Here's how the part is built. I have some questions about the finished solid (model axes, mm). A direction names the side the tool comes from. Give positions to 0.01 mm unless a question says otherwise; leave off trailing zeros. Order: outer loops, then holes, each group sorted by start corner. A loop starts at its lowest first (then second) coordinate and runs counter-clockwise, first axis right, second up.
from build123d import *

# Parameters (mm, degrees)
F0_R      = 3.1
F0_W      = 5.4
F0_H      = 6
F0_W_2    = 6
F0_H_2    = 5.4
F1_DEPTH  = 6
F2_DEPTH  = 10
F3_R      = 2
F4_SIZE   = 3.5
F1_FACE_R = 6.6
F5_DEPTH  = 2


with BuildPart() as f1:
    # F0 (on Top) → F1 (new body)
    with BuildSketch(Plane.XY):
        Polygon((-7.995946, 7.05), (-7.995946, 0), (-0.945946, 0), (-0.945946, 5.4), (5.054054, 5.4), (5.054054, 0), (12.104054, 0), (12.104054, 7.05), (6.704054, 7.05), (6.704054, 13.05), (12.104054, 13.05), (12.104054, 20.1), (5.054054, 20.1), (5.054054, 14.7), (-0.945946, 14.7), (-0.945946, 20.1), (-7.995946, 20.1), (-7.995946, 13.05), (-2.595946, 13.05), (-2.595946, 7.05), align=None)
        with Locations((2.054054, 10.05)):
            Circle(F0_R, mode=Mode.SUBTRACT)
        with Locations((9.404054, 10.05)):
            Rectangle(F0_W, F0_H)
        with Locations((-5.295946, 10.05)):
            Rectangle(F0_W, F0_H)
        with Locations((2.054054, 17.4)):
            Rectangle(F0_W_2, F0_H_2)
        with Locations((2.054054, 2.7)):
            Rectangle(F0_W_2, F0_H_2)
    extrude(amount=F1_DEPTH)

    # F0 (on Top) → F2 (join)
    with BuildSketch(Plane.XY):
        with Locations((2.054054, 17.4)):
            Rectangle(F0_W_2, F0_H_2)
        with Locations((-5.295946, 10.05)):
            Rectangle(F0_W, F0_H)
        with Locations((2.054054, 2.7)):
            Rectangle(F0_W_2, F0_H_2)
        with Locations((9.404054, 10.05)):
            Rectangle(F0_W, F0_H)
    extrude(amount=F2_DEPTH)

    # F3
    f3_edges = [f1.edges().sort_by_distance(p)[0] for p in [
        (-7.995946, 0, 3),
        (12.104054, 0, 3),
        (12.104054, 20.1, 3),
        (-7.995946, 20.1, 3),
    ]]
    fillet(f3_edges, radius=F3_R)

    # F4
    f4_edges = [f1.edges().sort_by_distance(p)[0] for p in [
        (-1.045946, 10.05, 0),
    ]]
    chamfer(f4_edges, length=F4_SIZE)

    # F1_face (on face) → F5 (join)
    with BuildSketch(Plane(origin=(2.054054, 10.05, 0), x_dir=(1, 0, 0), z_dir=(0, 0, -1))):
        with BuildLine():
            Line((-8.05, -10.05), (8.05, -10.05))
            ThreePointArc((8.05, -10.05), (9.464214, -9.464214), (10.05, -8.05))
            Line((10.05, -8.05), (10.05, 8.05))
            ThreePointArc((10.05, 8.05), (9.464214, 9.464214), (8.05, 10.05))
            Line((8.05, 10.05), (-8.05, 10.05))
            ThreePointArc((-8.05, 10.05), (-9.464214, 9.464214), (-10.05, 8.05))
            Line((-10.05, 8.05), (-10.05, -8.05))
            ThreePointArc((-10.05, -8.05), (-9.464214, -9.464214), (-8.05, -10.05))
        make_face()
        Circle(F1_FACE_R, mode=Mode.SUBTRACT)
    extrude(amount=F5_DEPTH)


solid = f1.part
Q1. I'm going to push flat-ended pins straight in: P1, Ø1.5, axis at x = 7, z = 7, coming from the -Y side; P2, Ø7, axis at x = 2.05, y = 10.05, coming from the -Z side; P3, Ø2, axis at x = -0.5, y = 10, coming from the -Z side. Where does each tip first touch, or does it pass through?
Filled sheet:
P1: stops at y = 7.05
P2: stops at z = 3.1
P3: stops at z = 3.05
Q2. If we section it at D-D on x = 11: List the corners of the cut face in (y, z) for me.
Filled sheet:
outline: (0.21, -2) - (19.89, -2) - (19.89, 6) - (13.05, 6) - (13.05, 10) - (7.05, 10) - (7.05, 6) - (0.21, 6) - close
Q3. Thinking about a two-plate mould opening in Y: for faces 5 (the face through (-0.946, 3, 8)), 6 (the face through (0.623, 16.493, -0.986)), 7 (the face through (2, 0, 3)), which applies, released by +Y, released by -Y, zero draft, split by the parting line, or undercut?
Filled sheet:
face 5: zero draft
face 6: undercut
face 7: released by -Y
Q4. For faces 1 (the face through (-0.946, 17, 8)), 2 (the face through (6.704, 10, 8)), 3 (the face through (5.054, 17, 8)), 4 (the face through (9, 7.05, 8)), which set-ups out of +Z, -Z, +X, -X, +Y, -Y let a thin tool reach every point of the face, with its end or its side?
Filled sheet:
face 1: +Z, -X, +Y, -Y
face 2: +Z, +Y, -Y
face 3: +Z, +X, +Y, -Y
face 4: +Z, +X, -X, -Y
Q5. If we section it at C-C on z = 6.5: List the corners of the cut face in (x, y) for me.
Filled sheet:
outline: (-8, 7.05) - (-2.6, 7.05) - (-2.6, 13.05) - (-8, 13.05) - close; (-0.95, 0) - (5.05, 0) - (5.05, 5.4) - (-0.95, 5.4) - close; (-0.95, 14.7) - (5.05, 14.7) - (5.05, 20.1) - (-0.95, 20.1) - close; (6.7, 7.05) - (12.1, 7.05) - (12.1, 13.05) - (6.7, 13.05) - close
Q6. If we section it at B-B on y = 10.05: List the corners of the cut face in (x, z) for me, plus the area to 3 significant figures.
Filled sheet:
outline: (-8, -2) - (-4.55, -2) - (-4.55, 0) - (-1.05, 3.5) - (-1.05, 6) - (-2.6, 6) - (-2.6, 10) - (-8, 10) - close; (5.15, 3.5) - (8.65, 0) - (8.65, -2) - (12.1, -2) - (12.1, 10) - (6.7, 10) - (6.7, 6) - (5.15, 6) - close
area: 128 mm2
Q7. If we section it at A-A on z = -0.5: List the corners of the cut face in (x, y) for me, plus the area to 3 significant figures.
Filled sheet:
outline: (-8, 2) arc R2 ccw to (-6, 0) - (10.1, 0) arc R2 ccw to (12.1, 2) - (12.1, 18.1) arc R2 ccw to (10.1, 20.1) - (-6, 20.1) arc R2 ccw to (-8, 18.1) - close; hole circle Ø13.2 at (2.05, 10.05)
area: 264 mm2
Q8. I need wall thicknesses on L1, parallel to Y at x = 1.5, z = 8.5; L2, parallel to X at y = 12.5, z = 7.75; L3, parallel to Z at x = -5, y = 16.75. Which ranges of each line are inside material? Lowest first, please.
Filled sheet:
L1: y = 0 to 5.4, 14.7 to 20.1
L2: x = -8 to -2.6, 6.7 to 12.1
L3: z = -2 to 6
